Design review of the part built by this model. Coordinates are the model's own, in mm. A direction names the side the tool comes from. Coordinates: 2 decimals unless noted, no trailing zeros. Write each loop counter-clockwise with the first axis right and the second up, starting at its lowest first coordinate (ties: lowest second). Pieces come first, ordered by that corner, then holes.
```python
from build123d import *

# Parameters (mm, degrees)
SKETCH1_W           = 100
SKETCH1_H           = 18
SKETCH1_R           = 4
BOSS_EXTRUDE1_DEPTH = 20
SKETCH2_W           = 50
SKETCH2_H           = 25
BOSS_EXTRUDE2_DEPTH = 15


with BuildPart() as part:
    # Sketch1 → Boss-Extrude1 (new body)
    with BuildSketch(Plane.XY):
        Rectangle(SKETCH1_W, SKETCH1_H)
        Circle(SKETCH1_R, mode=Mode.SUBTRACT)
    extrude(amount=BOSS_EXTRUDE1_DEPTH)

    # Sketch2 → Boss-Extrude2 (add, symmetric)
    with BuildSketch(Plane.XY.offset(10)):
        with Locations((45, 0)):
            Rectangle(SKETCH2_W, SKETCH2_H)
    extrude(amount=BOSS_EXTRUDE2_DEPTH, both=True)


solid = part.part
```
(1) Consider section A-A (y = 0). Give the boundary of the cut face in (x, z), plus the area to 3 significant figures.
(2) Mouldability with a two-part tool opening along X and no side actions: class faces 1 (the cylindrical face through (-0.867, -3.905, 9.86)), 2 (the flat face through (-50, 0, 10)), 3 (the flat face through (70, 0, 10)), 4 (the flat face through (-15, -9, 10)) as +X half, -X half, draft (parallel to the pull), parting line (faces both ways), or undercut.
(3) Consider section C-C (z = 18). Give the boundary of the cut face in (x, y), plus the area to 3 significant figures.
(4) For faces 5 (the flat face through (-15, 9, 10)), 6 (the flat face through (-15, 0, 0)), 7 (the flat face through (45, -12.5, 10)), 8 (the flat face through (-15, 0, 20)), list the 3-axis set-ups (+Z, -Z, +X, -X, +Y, -Y) from which the entire face can be reached by the end or side of a thin tool; tool diameter is ignored.
(5) Wall thickness on line 1 (Y direction, x = 0, z = 4.5); line 2 (Z direction, x = 5.5, y = 3); line 3 (X direction, y = 1.5, z = -1.5): over which ranges is each line inside the solid? List them lowest first.
(6) Insertion check: pin 1 Ø14.5 at (x, y) = (-9.5, -3) entering from +Z; pin 2 Ø6 at (x, z) = (-31, 11.5) entering from -Y; pin 3 Ø5 at (x, z) = (3.5, 10) entering from +Y. Each pin has a flat end and moves straight along its axis. Give the tip position at first contact, or say it passes through.
(7) Consider section B-B (x = 0). Give the boundary of the cut face in (y, z).
(8) Consider section D-D (y = -5.75). Give the boundary of the cut face in (x, z).
Results:
1. outline: (-50, 0) - (-4, 0) - (-4, 20) - (-50, 20) - close; (4, 0) - (20, 0) - (20, -5) - (70, -5) - (70, 25) - (20, 25) - (20, 20) - (4, 20) - close
1. area: 2,740 mm2
2. face 1: undercut
2. face 2: -X half
2. face 3: +X half
2. face 4: draft
3. outline: (-50, -9) - (20, -9) - (20, -12.5) - (70, -12.5) - (70, 12.5) - (20, 12.5) - (20, 9) - (-50, 9) - close; hole circle Ø8 at (0, 0)
3. area: 2,460 mm2
4. face 5: +Z, -Z, -X, +Y
4. face 6: -Z, -X, +Y, -Y
4. face 7: +Z, -Z, +X, -X, -Y
4. face 8: +Z, -X, +Y, -Y
5. line 1: y = -9 to -4, 4 to 9
5. line 2: z = 0 to 20
5. line 3: x = 20 to 70
6. pin 1: stops at z = 20
6. pin 2: stops at y = -9
6. pin 3: stops at y = 9
7. outline: (-9, 0) - (-4, 0) - (-4, 20) - (-9, 20) - close; (4, 0) - (9, 0) - (9, 20) - (4, 20) - close
8. outline: (-50, 0) - (20, 0) - (20, -5) - (70, -5) - (70, 25) - (20, 25) - (20, 20) - (-50, 20) - close
